from build123d import *

# Parameters (mm, degrees)
F0_W     = 80
F0_H     = 5
F1_DEPTH = 100
F2_R     = 3
F3_DEPTH = 25
F4_R     = 1.5
F5_DEPTH = 25
F6_R     = 2
F7_DEPTH = 25
F8_R     = 2
F9_DEPTH = 25


with BuildPart() as f1:
    # F0 (on Top) → F1 (new body)
    with BuildSketch(Plane.XY):
        with Locations((40, 2.5)):
            Rectangle(F0_W, F0_H)
    extrude(amount=F1_DEPTH)

    # F2 (on face) → F3 (cut)
    with BuildSketch(Plane(origin=(0, 5, 0), x_dir=(-1, 0, 0), z_dir=(0, 1, 0))):
        with Locations((-5, 83)):
            Circle(F2_R)
        with Locations((-75, 83)):
            Circle(F2_R)
    extrude(amount=-F3_DEPTH, mode=Mode.SUBTRACT)

    # F4 (on face) → F5 (cut)
    with BuildSketch(Plane.XZ):
        with Locations((45, 50)):
            Circle(F4_R)
        with Locations((35, 50)):
            Circle(F4_R)
    extrude(amount=-F5_DEPTH, mode=Mode.SUBTRACT)

    # F6 (on face) → F7 (cut)
    with BuildSketch(Plane.XZ):
        with Locations((75, 95)):
            Circle(F6_R)
        with Locations((55, 95)):
            Circle(F6_R)
    extrude(amount=-F7_DEPTH, mode=Mode.SUBTRACT)

    # F8 (on face) → F9 (cut)
    with BuildSketch(Plane.XZ):
        with Locations((33, 58)):
            Circle(F8_R)
        with Locations((47, 58)):
            Circle(F8_R)
    extrude(amount=-F9_DEPTH, mode=Mode.SUBTRACT)


solid = f1.part
Could you check a few things on this model? Use its own coordinates, in mm. Round coordinates to 2 decimals unless told otherwise and drop trailing zeros. Order: outer loops, then holes, each group sorted by start corner. A loop starts at its lowest first (then second) coordinate and runs counter-clockwise, first axis right, second up.
(1) If we mould it in two halves opening along X, with no side actions, what happens to faces 1 (the cylindrical face through (76.075, 2.465, 96.686)), 2 (the flat face through (39, 3, 100)), 3 (the flat face through (0, 2, 49))? For each: released by +X, released by -X, zero draft, split by the parting line, or undercut.
Response values:
face 1: undercut
face 2: zero draft
face 3: released by -X
(2) Imagine slicing it at B-B (x = 55). Write out the boundary of the cut face in (y, z), plus the area to 3 significant figures.
Response values:
outline: (0, 0) - (5, 0) - (5, 93) - (0, 93) - close; (0, 97) - (5, 97) - (5, 100) - (0, 100) - close
area: 480 mm2
(3) Imagine slicing it at A-A (z = 83). Write out the boundary of the cut face in (x, y), plus the area to 3 significant figures.
Response values:
outline: (0, 0) - (2, 0) - (2, 5) - (0, 5) - close; (8, 0) - (72, 0) - (72, 5) - (8, 5) - close; (78, 0) - (80, 0) - (80, 5) - (78, 5) - close
area: 340 mm2
(4) Imagine slicing it at D-D (x = 75). Write out the boundary of the cut face in (y, z).
Response values:
outline: (0, 0) - (5, 0) - (5, 80) - (0, 80) - close; (0, 86) - (5, 86) - (5, 93) - (0, 93) - close; (0, 97) - (5, 97) - (5, 100) - (0, 100) - close
(5) I'm going to push a flat-ended pin straight in: pin 1 (2.5 mm diameter, centred on x = 47, z = 58, fed in from +Y). Where does the tip first touch, or does it pass through?
Response values:
pin 1: passes through
(6) Please list where these lines run through material, in increasing order: line 1 along Z through (x, y) = (75, 2.8); line 2 along Z through (x, y) = (55, 2); line 3 along Z through (x, y) = (33, 2.8).
Response values:
line 1: z = 0 to 80, 86 to 93, 97 to 100
line 2: z = 0 to 93, 97 to 100
line 3: z = 0 to 56, 60 to 100
(7) Imagine slicing it at C-C (y = 3.55). Count the separate pieces of the cut face and the enclosed holes in it, plus the area to 3 significant figures.
Response values:
separate pieces: 1
enclosed holes: 8
area: 7,880 mm2
